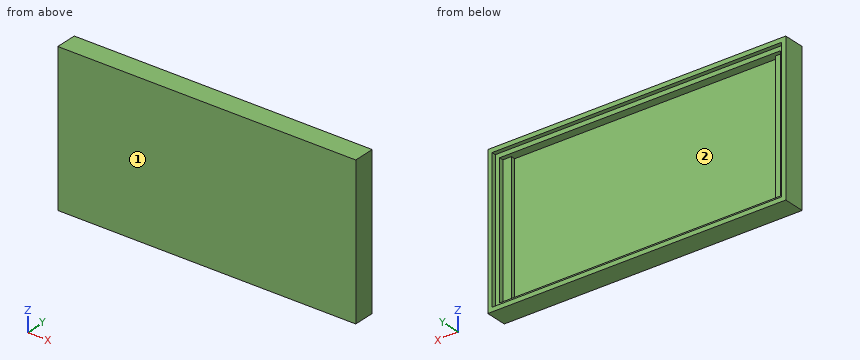
```python
from build123d import *

# Parameters (mm, degrees)
SKETCH1_W           = 70
SKETCH1_H           = 35
BOSS_EXTRUDE1_DEPTH = 2
SKETCH2_W           = 70
SKETCH2_H           = 35
SKETCH2_W_2         = 66
SKETCH2_H_2         = 31
BOSS_EXTRUDE2_DEPTH = 2
SKETCH3_W           = 2
SKETCH3_H           = 31
BOSS_EXTRUDE3_DEPTH = 1
SKETCH4_W           = 70
SKETCH4_H           = 35
SKETCH4_W_2         = 68
SKETCH4_H_2         = 33
BOSS_EXTRUDE4_DEPTH = 1


with BuildPart() as part:
    # Sketch1 → Boss-Extrude1 (new body)
    with BuildSketch(Plane(origin=(0, 0, 0), x_dir=(1, 0, 0), z_dir=(0, 1, 0))):
        with Locations((33, 15.5)):
            Rectangle(SKETCH1_W, SKETCH1_H)
    extrude(amount=BOSS_EXTRUDE1_DEPTH)

    # Sketch2 → Boss-Extrude2 (add)
    with BuildSketch(Plane(origin=(0, 2, 0), x_dir=(1, 0, 0), z_dir=(0, 1, 0))):
        with Locations((33, 15.5)):
            Rectangle(SKETCH2_W, SKETCH2_H)
        with Locations((33, 15.5)):
            Rectangle(SKETCH2_W_2, SKETCH2_H_2, mode=Mode.SUBTRACT)
    extrude(amount=BOSS_EXTRUDE2_DEPTH)

    # Sketch3 → Boss-Extrude3 (add)
    with BuildSketch(Plane(origin=(0, 2, 0), x_dir=(1, 0, 0), z_dir=(0, 1, 0))):
        with Locations((1, 15.5)):
            Rectangle(SKETCH3_W, SKETCH3_H)
        with Locations((65, 15.5)):
            Rectangle(SKETCH3_W, SKETCH3_H)
    extrude(amount=BOSS_EXTRUDE3_DEPTH)

    # Sketch4 → Boss-Extrude4 (add)
    with BuildSketch(Plane(origin=(0, 4, 0), x_dir=(1, 0, 0), z_dir=(0, 1, 0))):
        with Locations((33, 15.5)):
            Rectangle(SKETCH4_W, SKETCH4_H)
        with Locations((33, 15.5)):
            Rectangle(SKETCH4_W_2, SKETCH4_H_2, mode=Mode.SUBTRACT)
    extrude(amount=BOSS_EXTRUDE4_DEPTH)


solid = part.part
```
CAD build for the part. Positions are in the model's coordinates, mm. Face numbers are marked on the shaded views. A direction names the side the tool comes from. Give positions to 0.01 mm unless a question says otherwise; leave off trailing zeros. Order: outer loops, then holes, each group sorted by start corner. A loop starts at its lowest first (then second) coordinate and runs counter-clockwise, first axis right, second up.
(1) Saw through at B-B, the plane x = 61.5. Give the cut face in (y, z), then the cut area to 3 significant figures.
(2) Flat gauge pins, fed straight in: pin 1 (0.6 mm diameter, centred on x = 1, z = -20.5, fed in from +Y); pin 2 (1 mm diameter, centred on x = 41.5, z = -28.5, fed in from -Y); pin 3 (6 mm diameter, centred on x = 26, z = -2.5, fed in from +Y). Where does each tip first touch, or does it go through?
(3) Drill centre lines: L1, parallel to Z at x = 10.5, y = 4.3; L2, parallel to X at y = 2.5, z = -23; L3, parallel to Z at x = 33, y = 3.3. Where is each one in solid material? Low to high.
(4) Tool access for the marked faces 1 and 2: list every direction of +Z, -Z, +X, -X, +Y, -Y with a clear straight run to the whole face (end or side of a thin tool).
(5) Saw through at A-A, the plane z = -9.5. Give the cut face in (x, y).
Results found:
1. outline: (0, -33) - (5, -33) - (5, -32) - (4, -32) - (4, -31) - (2, -31) - (2, 0) - (4, 0) - (4, 1) - (5, 1) - (5, 2) - (0, 2) - close
1. area: 80.0 mm2
2. pin 1: stops at y = 3
2. pin 2: stops at y = 0
2. pin 3: stops at y = 4
3. L1: z = -33 to -32, 1 to 2
3. L2: x = -2 to 2, 64 to 68
3. L3: z = -33 to -31, 0 to 2
4. face 1: +Z, -Z, +X, -X, -Y
4. face 2: +Y
5. outline: (-2, 0) - (68, 0) - (68, 5) - (67, 5) - (67, 4) - (66, 4) - (66, 3) - (64, 3) - (64, 2) - (2, 2) - (2, 3) - (0, 3) - (0, 4) - (-1, 4) - (-1, 5) - (-2, 5) - close
